Can you work these out from the model? Positions are in its coordinate system, mm. Face numbers are marked on the shaded views. A direction names the side the tool comes from. Round coordinates to 2 decimals unless told otherwise and drop trailing zeros. Order: outer loops, then holes, each group sorted by start corner. A loop starts at its lowest first (then second) coordinate and runs counter-clockwise, first axis right, second up.
Q1. Will these pins go through, and if not, where does the flat tip stop? P1, Ø12, axis at x = 15, y = 4, coming from the +Z side; P2, Ø1, axis at x = -27.5, z = 18.5, coming from the +Y side; P3, Ø8, axis at x = -65.5, z = 19.5, coming from the +Y side; P4, Ø16, axis at y = 4, z = 3, coming from the +X side.
Q2. If we section it at A-A (x = -72.5): Please give me the cut outline in (y, z), plus the area to 3 significant figures.
Q3. We'd pull the mould along X, two halves only. Please class the marked faces 1, 2 and 3: pulls with the +X half, pulls with the -X half, needs draft (parallel to the pull), parting line crosses it, or undercut.
Q4. If we section it at D-D (z = 25.5): Please give me the cut outline in (x, y), plus the area to 3 significant figures.
Q5. If I drill on line 1 (Y direction, x = -72.5, z = 11.75); line 2 (X direction, y = 1, z = 18); line 3 (Z direction, x = -8, y = -11), over which ranges is the centre line in solid material (lowest first)?
Q6. If we section it at B-B (z = 9): Please give me the cut outline in (x, y).
Q7. For the marked faces 4, 5 and 6, which set-ups out of +Z, -Z, +X, -X, +Y, -Y let a thin tool reach every point of the face, with its end or its side?
Q8. If we section it at C-C (y = 0): Please give me the cut outline in (x, z).
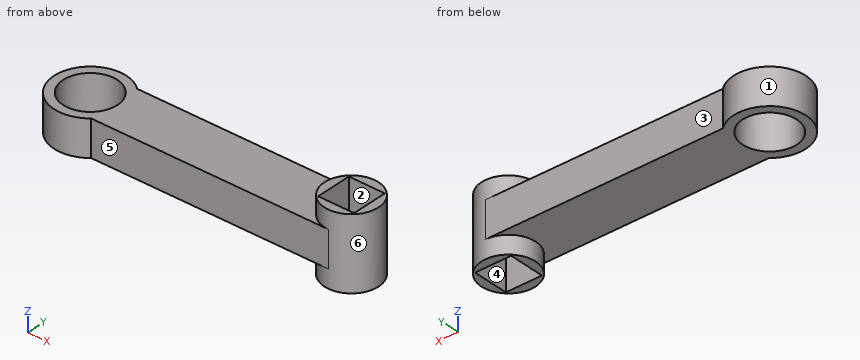
from build123d import *

# Parameters (mm, degrees)
SKETCH1_R           = 15
BOSS_EXTRUDE2_DEPTH = 20
SKETCH3_R           = 15
BOSS_EXTRUDE3_DEPTH = 10
BOSS_EXTRUDE4_START = 10
SKETCH5_R           = 15
BOSS_EXTRUDE4_DEPTH = 10
SKETCH6_W           = 20
SKETCH6_H           = 20
CUT_EXTRUDE1_DEPTH  = 50


with BuildPart() as part:
    # Sketch1 → Boss-Extrude2 (new body)
    with BuildSketch(Plane.XY):
        with BuildLine():
            Line((72.5, -15), (-59.271243445, -15))
            ThreePointArc((-59.271243445, -15), (-92.5, 0), (-59.271243445, 15))
            Line((-59.271243445, 15), (72.5, 15))
            ThreePointArc((72.5, 15), (87.5, 0), (72.5, -15))
        make_face()
        with Locations((-72.5, 0)):
            Circle(SKETCH1_R, mode=Mode.SUBTRACT)
    extrude(amount=BOSS_EXTRUDE2_DEPTH)

    # Sketch3 → Boss-Extrude3 (add)
    with BuildSketch(Plane.XY.offset(20)):
        with Locations(Location((72.5, 0, 0), (0, 0, 90))):
            Circle(SKETCH3_R)
    extrude(amount=BOSS_EXTRUDE3_DEPTH)

    # Sketch5 → Boss-Extrude4 (add)
    with BuildSketch(Plane(origin=(0, 0, 0), x_dir=(-1, 0, 0), z_dir=(0, 0, -1)).offset(BOSS_EXTRUDE4_START)):
        with Locations((-72.5, 0)):
            Circle(SKETCH5_R)
    extrude(amount=-BOSS_EXTRUDE4_DEPTH)

    # Sketch6 → Cut-Extrude1 (cut)
    with BuildSketch(Plane(origin=(0, 0, -10), x_dir=(-1, 0, 0), z_dir=(0, 0, -1))):
        with Locations((-72.5, 0)):
            Rectangle(SKETCH6_W, SKETCH6_H)
    extrude(amount=-CUT_EXTRUDE1_DEPTH, mode=Mode.SUBTRACT)


solid = part.part
Solution:
1. P1: stops at z = 20
1. P2: stops at y = 15
1. P3: stops at y = 19.77
1. P4: stops at x = 87.5
2. outline: (-20, 0) - (-15, 0) - (-15, 20) - (-20, 20) - close; (15, 0) - (20, 0) - (20, 20) - (15, 20) - close
2. area: 200 mm2
3. face 1: parting line crosses it
3. face 2: undercut
3. face 3: needs draft
4. outline: circle Ø30 at (72.5, 0); hole (62.5, -10) - (82.5, -10) - (82.5, 10) - (62.5, 10) - close
4. area: 307 mm2
5. line 1: y = -20 to -15, 15 to 20
5. line 2: x = -92.47 to -87.47, -57.53 to 62.5, 82.5 to 87.47
5. line 3: z = 0 to 20
6. outline: (-59.27, -15) - (72.5, -15) arc R15 ccw to (72.5, 15) - (-59.27, 15) arc R20 ccw (long way) to start; hole circle Ø30 at (-72.5, 0); hole (62.5, -10) - (82.5, -10) - (82.5, 10) - (62.5, 10) - close
7. face 4: +Z, -Z
7. face 5: +Z, -Z, +X, -Y
7. face 6: none
8. outline: (-92.5, 0) - (-87.5, 0) - (-87.5, 20) - (-92.5, 20) - close; (-57.5, 0) - (57.5, 0) - (57.5, -10) - (62.5, -10) - (62.5, 30) - (57.5, 30) - (57.5, 20) - (-57.5, 20) - close; (82.5, -10) - (87.5, -10) - (87.5, 30) - (82.5, 30) - close
